```python
from build123d import *

# Parameters (mm, degrees)
AUFSATZ_LINEAR_AUSTRAGEN1_DEPTH = 4
SKIZZE4_R                       = 1.5
SCHNITT_LINEAR_AUSTRAGEN4_DEPTH = 4


with BuildPart() as part:
    # Skizze2 → Aufsatz-Linear austragen1 (new body)
    with BuildSketch(Plane(origin=(0, 0, 0), x_dir=(1, 0, 0), z_dir=(0, 1, 0))):
        with BuildLine():
            Line((26.970562748, 26.970562748), (17.071067812, 17.071067812))
            ThreePointArc((17.071067812, 17.071067812), (14.903340299, 6.173165676), (24.142135624, 0))
            Line((24.142135624, 0), (43.941125497, 0))
            ThreePointArc((43.941125497, 0), (53.179920822, 6.173165676), (51.012193309, 17.071067812))
            Line((51.012193309, 17.071067812), (41.112698372, 26.970562748))
            ThreePointArc((41.112698372, 26.970562748), (34.04163056, 29.899494937), (26.970562748, 26.970562748))
        make_face()
    extrude(amount=AUFSATZ_LINEAR_AUSTRAGEN1_DEPTH)

    # Skizze4 → Schnitt-Linear austragen4 (cut)
    with BuildSketch(Plane(origin=(0, 0, 0), x_dir=(1, 0, 0), z_dir=(0, 1, 0))):
        with Locations(Location((21.54163056, 8.754981608, 0), (0, 0, 90))):
            Circle(SKIZZE4_R)
        with Locations(Location((46.54163056, 8.754981608, 0), (0, 0, 90))):
            Circle(SKIZZE4_R)
    extrude(amount=SCHNITT_LINEAR_AUSTRAGEN4_DEPTH, mode=Mode.SUBTRACT)


solid = part.part
```
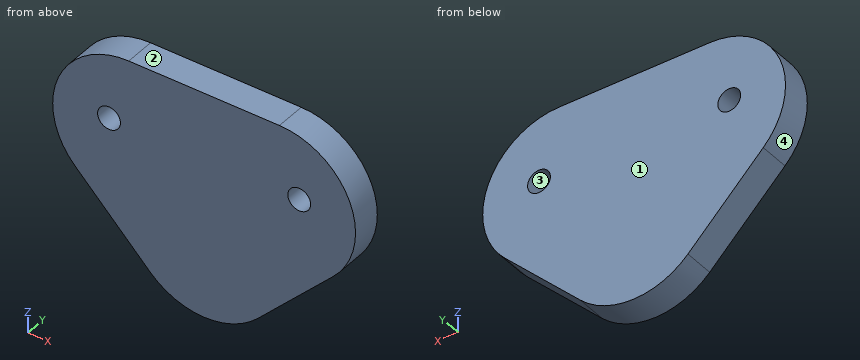
Design review of the part built by this model. Coordinates are the model's own, in mm. Face numbers are marked on the shaded views. Coordinates: 2 decimals unless noted, no trailing zeros. Order: outer loops, then holes, each group sorted by start corner. A loop starts at its lowest first (then second) coordinate and runs counter-clockwise, first axis right, second up. Notation, with made-up numbers: (43, 14) -> (59, 14) arc R25 ccw to (59, 50) -> close; hole circle Ø3 at (-18, -17.5). An arc over 180 degrees is marked (long way). One line per item, written item: value. Start each with the question number.
Q1. Insertion check: pin 1 Ø2 at (y, z) = (3.5, -17.5) entering from +X. The pin has a flat end and moves straight along its axis. Give the tip position at first contact, or say it passes through.
Q2. Take a section at B-B, the plane y = 0.9. State the section outline as (x, z) points, then the cut area to 3 significant figures.
Q3. Take a section at D-D, the plane x = 39.5. State the section outline as (y, z) points, then the cut area to 3 significant figures.
Q4. Mouldability with a two-part tool opening along Z and no side actions: class the marked faces 1, 2, 3 and 4 as pulls with the +Z half, pulls with the -Z half, needs draft (parallel to the pull), parting line crosses it, or undercut.
Q5. For probe 1 along X at (y, z) = (3.5, -9); probe 2 along X at (y, z) = (2.8, -2.75); probe 3 along Z at (x, y) = (33, 2.65), list the stretches that pass through material, from the lowest coordinate up.
Q6. Take a section at C-C, the plane z = -15. State the section outline as (x, y) points, then the cut area to 3 significant figures.
Q7. Take a section at A-A, the plane x = 45.5. State the section outline as (y, z) points, then the cut area to 3 significant figures.
Values follow:
1. pin 1: stops at x = 51.54
2. outline: (17.07, -17.07) -> (26.97, -26.97) arc R10 ccw to (41.11, -26.97) -> (51.01, -17.07) arc R10 ccw to (43.94, 0) -> (24.14, 0) arc R10 ccw to start; hole circle Ø3 at (21.54, -8.75); hole circle Ø3 at (46.54, -8.75)
2. area: 876 mm2
3. outline: (0, -28.28) -> (4, -28.28) -> (4, 0) -> (0, 0) -> close
3. area: 113 mm2
4. face 1: needs draft
4. face 2: pulls with the +Z half
4. face 3: undercut
4. face 4: parting line crosses it
5. probe 1: x = 14.19 to 20.06, 23.02 to 45.06, 48.02 to 53.89
5. probe 2: x = 17.25 to 50.83
5. probe 3: z = -29.85 to 0
6. outline: (15.48, 0) -> (52.6, 0) -> (52.6, 4) -> (15.48, 4) -> close
6. area: 148 mm2
7. outline: (0, -22.58) -> (4, -22.58) -> (4, -9.83) -> (0, -9.83) -> close; (0, -7.68) -> (4, -7.68) -> (4, -0.12) -> (0, -0.12) -> close
7. area: 81.2 mm2
